Read the model definition and answer for the solid it produces. Units are mm, in the model's axes. A direction names the side the tool comes from. Coordinates: 2 decimals unless noted, no trailing zeros. Loops run counter-clockwise (first coordinate to the right, second up) from the corner with the lowest first, then second, coordinate; pieces in that order, holes last. Notation, with made-up numbers: (29, 66.25) -> (83, 66.25) arc R8 cw to (83, 70.25) -> close; hole circle Ø3 at (35, 52). An arc over 180 degrees is marked (long way). One line per question, with ' | ' between items. Start each with the question number.
```python
from build123d import *

# Parameters (mm, degrees)
F0_W     = 113.5605871677
F0_H     = 73.2877403498
F1_DEPTH = 254
F2_T     = -0.254
F7_DEPTH = 23.6716698855


with BuildPart() as f1:
    # F0 (on Top) → F1 (new body)
    with BuildSketch(Plane.XY):
        with Locations((-56.7802935839, 36.6438701749)):
            Rectangle(F0_W, F0_H)
    extrude(amount=F1_DEPTH)

    # F2
    f2_openings = [f1.faces().sort_by_distance(p)[0] for p in [
        (0, 36.64387, 127),
    ]]
    offset(amount=F2_T, openings=f2_openings)


with BuildPart() as f5:
    # F4 (on Top) → F5 (revolve)
    with BuildSketch(Plane.XY):
        Polygon((128.8485527039, 0), (0, 0), (0, -32.9870469868), (12.1806450188, -32.9870469868), (12.1806450188, -14.4056975842), (18.5923762619, -14.4056975842), (18.5923762619, -32.9870469868), (27.2095799446, -32.9870469868), (27.2095799446, -23.6716698855), (67.0536756516, -23.6716698855), (104.2113080621, -58.7185546756), (128.8485527039, -40.4047630727), align=None)
    revolve(axis=Axis((0, -16.4935234934, 0), (0, 1, 0)))

    # F6 (on face) → F7 (cut, through all)
    with BuildSketch(Plane.XZ.offset(23.6716698855)):
        with BuildLine():
            ThreePointArc((26.7019728343, 53.911552779), (28.0869530427, 58.521028427), (25.0041931016, 62.2172463688))
            ThreePointArc((25.0041931016, 62.2172463688), (16.1643801545, 65.0761725411), (7.0142513747, 66.6857983085))
            ThreePointArc((7.0142513747, 66.6857983085), (2.1012058316, 65.0897727595), (0, 60.3706363857))
            Line((0, 60.3706363857), (0, 36.4077336173))
            ThreePointArc((0, 36.4077336173), (2.3519761227, 32.8877525984), (6.5040768363, 33.7136567809))
            Line((6.5040768363, 33.7136567809), (26.7019728343, 53.911552779))
        make_face()
        with BuildLine():
            ThreePointArc((41.3796193581, -52.7628896115), (48.2754285244, -46.5368501208), (54.2444697194, -39.4174190332))
            ThreePointArc((54.2444697194, -39.4174190332), (55.3187938204, -34.3645840085), (52.2825047526, -30.1853181928))
            Line((52.2825047526, -30.1853181928), (31.5300222068, -18.2038668086))
            ThreePointArc((31.5300222068, -18.2038668086), (27.3056411622, -18.4807473705), (25.9448448086, -22.4895241589))
            Line((25.9448448086, -22.4895241589), (33.3377878469, -50.0803631952))
            ThreePointArc((33.3377878469, -50.0803631952), (36.6372207521, -53.5845290634), (41.3796193581, -52.7628896115))
        make_face()
        with BuildLine():
            ThreePointArc((-60.0397606812, -3.8311895838), (-64.7241737948, -4.9364993636), (-66.3838124597, -9.4543567573))
            ThreePointArc((-66.3838124597, -9.4543567573), (-64.4398086789, -18.5393224203), (-61.2587210941, -27.2683792752))
            ThreePointArc((-61.2587210941, -27.2683792752), (-57.4199996521, -30.725188751), (-52.2825047526, -30.1853181928))
            Line((-52.2825047526, -30.1853181928), (-31.5300222068, -18.2038668086))
            ThreePointArc((-31.5300222068, -18.2038668086), (-29.6576172849, -14.4070052278), (-32.4489216449, -11.224132622))
            Line((-32.4489216449, -11.224132622), (-60.0397606812, -3.8311895838))
        make_face()
    extrude(amount=-F7_DEPTH, mode=Mode.SUBTRACT)


solid = f5.part
```
(1) Find the intervals of material crossed by probe 1 along X at (y, z) = (-22, 0); probe 2 along Z at (x, y) = (0, -25.25); probe 3 along X at (y, z) = (-29, -19), in increasing order. Write a range as from..to.
(2) Section B-B on z = 0 is taken. Write down the section's boundary in (x, y).
(3) Section C-C on y = -37 is taken. Write down the section's boundary in (x, z).
(4) Each of these flat-tipped pins is pushed along its axis until it touches: pin 1 Ø12 at (y, z) = (-49.5, -81) entering from +X; pin 2 Ø10 at (x, y) = (79, -39.5) entering from +Z; pin 3 Ø1.5 at (x, z) = (-11, -59) entering from -Y. Where does it stop, or does it pass through?
(5) A tool of negligible diameter and unlimited length cuts with its end or side. For faces 1 (the flat face through (-29, -23.672, -1)), 2 (the cylindrical face through (48.185, -12.002, -46.63)), from which of +Z, -Z, +X, -X, +Y, -Y can it reach the whole face along a straight path? Write none if from no direction.
(6) Section A-A on y = -19.5 is taken. Write down the section's boundary in (x, z).
(7) Determine the mould class of faces 3 (the flat face through (-2, 0, -2)), 4 (the conical face through (-22.93, -57.57, 103.24)), 5 (the flat face through (0, -12, 49)), 6 (the flat face through (16.46, -12, 43.67)) for opening direction X: +X half, -X half, draft (parallel to the pull), parting line (faces both ways), or undercut.
Working result:
1) probe 1: x = -128.85..-18.59, -12.18..12.18, 18.59..128.85 | probe 2: z = -128.85..-68.73, -27.21..-18.59, -12.18..12.18, 18.59..27.21, 68.73..128.85 | probe 3: x = -127.44..-70.18, -19.48..19.48, 70.18..127.44
2) outline: (-128.85, -40.4) -> (-104.21, -58.72) -> (-67.05, -23.67) -> (-27.21, -23.67) -> (-27.21, -32.99) -> (-18.59, -32.99) -> (-18.59, -14.41) -> (-12.18, -14.41) -> (-12.18, -32.99) -> (12.18, -32.99) -> (12.18, -14.41) -> (18.59, -14.41) -> (18.59, -32.99) -> (27.21, -32.99) -> (27.21, -23.67) -> (67.05, -23.67) -> (104.21, -58.72) -> (128.85, -40.4) -> (128.85, 0) -> (-128.85, 0) -> close
3) outline: circle Ø257.7 at (0, 0); hole circle Ø162.37 at (0, 0)
4) pin 1: stops at x = 95.92 | pin 2: stops at z = 105.48 | pin 3: stops at y = -23.67
5) face 1: -Y | face 2: +Y, -Y
6) outline: circle Ø257.7 at (0, 0); circle Ø24.36 at (0, 0); hole (-66.38, -9.45) arc R67.05 ccw to (-61.26, -27.27) arc R6.35 ccw to (-52.28, -30.19) -> (-31.53, -18.2) arc R3.81 ccw to (-32.45, -11.22) -> (-60.04, -3.83) arc R5.08 ccw to start; hole circle Ø37.18 at (0, 0); hole (0, 36.41) arc R3.81 ccw to (6.5, 33.71) -> (26.7, 53.91) arc R5.08 ccw to (25, 62.22) arc R67.05 ccw to (7.01, 66.69) arc R6.35 ccw to (0, 60.37) -> close; hole (25.94, -22.49) -> (33.34, -50.08) arc R5.08 ccw to (41.38, -52.76) arc R67.05 ccw to (54.24, -39.42) arc R6.35 ccw to (52.28, -30.19) -> (31.53, -18.2) arc R3.81 ccw to start
7) face 3: draft | face 4: parting line | face 5: undercut | face 6: undercut
